Build history of the part. All positions in model axes, mm. Face numbers are marked on the shaded views. A direction names the side the tool comes from. Round coordinates to 2 decimals unless told otherwise and drop trailing zeros. Write each loop counter-clockwise with the first axis right and the second up, starting at its lowest first coordinate (ties: lowest second). Pieces come first, ordered by that corner, then holes. Notation, with made-up numbers: (66.25, 73.25) -> (98.25, 73.25) arc R22 cw to (98.25, 82.25) -> close; hole circle Ø7 at (-14.75, 38.25). An arc over 180 degrees is marked (long way). Answer in a Markdown table with one row per item.
```python
from build123d import *

# Parameters (mm, degrees)
ESQUISSE1_R        = 0.8
ESQUISSE1_R_2      = 3
BOSS_EXTRU_1_DEPTH = 5


with BuildPart() as part:
    # Esquisse1 → Boss.-Extru.1 (new, symmetric)
    with BuildSketch(Plane.XY):
        with BuildLine():
            Line((-15, 13.5), (-15, -43.010256567))
            ThreePointArc((-15, -43.010256567), (-14.441599081, -46.305132406), (-12.828758641, -49.232035906))
            Line((-12.828758641, -49.232035906), (-12.171241359, -50.059378669))
            ThreePointArc((-12.171241359, -50.059378669), (-10.558400919, -52.986282168), (-10, -56.281158007))
            Line((-10, -56.281158007), (-10, -92.791414574))
            Line((-10, -92.791414574), (10, -92.791414574))
            Line((10, -92.791414574), (10, -56.281158007))
            ThreePointArc((10, -56.281158007), (10.558400919, -52.986282168), (12.171241359, -50.059378669))
            Line((12.171241359, -50.059378669), (12.828758641, -49.232035906))
            ThreePointArc((12.828758641, -49.232035906), (14.441599081, -46.305132406), (15, -43.010256567))
            Line((15, -43.010256567), (15, 13.5))
            ThreePointArc((15, 13.5), (0, 28.5), (-15, 13.5))
        make_face()
        with Locations((-0.005270268, 5.998754805)):
            Circle(ESQUISSE1_R, mode=Mode.SUBTRACT)
        with Locations((-7.505270268, 13.498754805)):
            Circle(ESQUISSE1_R, mode=Mode.SUBTRACT)
        with Locations((-0.005270268, 20.998754805)):
            Circle(ESQUISSE1_R, mode=Mode.SUBTRACT)
        with Locations((7.494729732, 13.498754805)):
            Circle(ESQUISSE1_R, mode=Mode.SUBTRACT)
        with Locations((-0.005270268, 13.498754805)):
            Circle(ESQUISSE1_R_2, mode=Mode.SUBTRACT)
    extrude(amount=BOSS_EXTRU_1_DEPTH, both=True)


solid = part.part
```
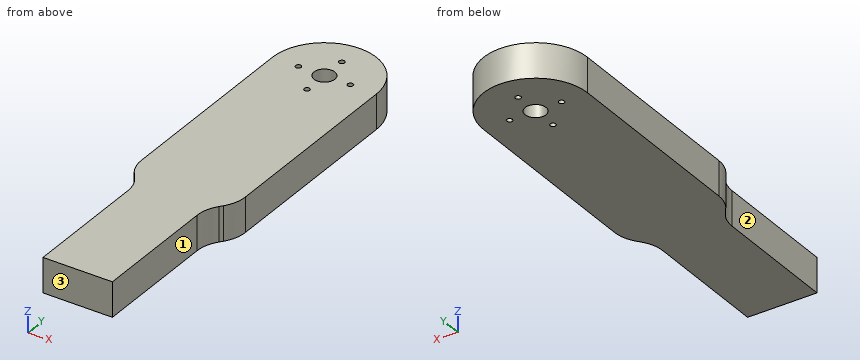
Q1. Saw through at A-A on z = -3.5. Write the cut outline in (x, y), plus the area to 3 significant figures.
A:
| item | result |
|---|---|
| outline | (-15, -43.01) arc R10 ccw to (-12.83, -49.23) -> (-12.17, -50.06) arc R10 cw to (-10, -56.28) -> (-10, -92.79) -> (10, -92.79) -> (10, -56.28) arc R10 cw to (12.17, -50.06) -> (12.83, -49.23) arc R10 ccw to (15, -43.01) -> (15, 13.5) arc R15 ccw to (-15, 13.5) -> close; hole circle Ø1.6 at (-7.51, 13.5); hole circle Ø6 at (-0.01, 13.5); hole circle Ø1.6 at (-0.01, 6); hole circle Ø1.6 at (-0.01, 21); hole circle Ø1.6 at (7.49, 13.5) |
| area | 3,070 mm² |
Q2. Drop flat-ended pins along their axis: P1, Ø5.5, axis at x = -0.01, y = 13.5, coming from the +Z side; P2, Ø2, axis at x = -12, z = -2.5, coming from the -Y side; P3, Ø2, axis at x = -0.01, y = 21, coming from the +Z side. Give the stop position or say it passes through.
A:
| item | result |
|---|---|
| P1 | through |
| P2 | y = -51.92 |
| P3 | z = 5 |
Q3. Which spindle directions (+Z, -Z, +X, -X, +Y, -Y) get a long thin tool onto all of the face, cutting with end or side? Do the marked faces 1, 2 and 3. Say none if no direction does.
A:
| item | result |
|---|---|
| face 1 | +Z, -Z, +X, -Y |
| face 2 | +Z, -Z, -X, -Y |
| face 3 | +Z, -Z, +X, -X, -Y |
Q4. Saw through at B-B on y = -59.5. Write the cut outline in (x, z).
A:
| item | result |
|---|---|
| outline | (-10, -5) -> (10, -5) -> (10, 5) -> (-10, 5) -> close |
Q5. Wall check: line 1 (Y direction, x = 8, z = 4.75); line 2 (Y direction, x = 0.5, z = 3.75); line 3 (Y direction, x = -2.5, z = 4). Give the ranges that are in metal, low to high. Write a range as [from, to].
A:
| item | result |
|---|---|
| line 1 | [-92.79, 12.88], [14.12, 26.19] |
| line 2 | [-92.79, 5.38], [6.62, 10.54], [16.46, 20.38], [21.62, 28.49] |
| line 3 | [-92.79, 11.83], [15.16, 28.29] |
